from build123d import *

# Parameters (mm, degrees)
SKETCH1_R           = 1
SKETCH1_R_2         = 1.5
BOSS_EXTRUDE1_DEPTH = 3
SKETCH2_R           = 1
CUT_EXTRUDE1_DEPTH  = 10


with BuildPart() as part:
    # Sketch1 → Boss-Extrude1 (new body)
    with BuildSketch(Plane.XY):
        with BuildLine():
            Line((56.489085284, -2.807723586), (56.489085284, -10.511796182))
            ThreePointArc((56.489085284, -10.511796182), (49.919430424, -21.212793876), (37.403860007, -20.196814652))
            ThreePointArc((37.403860007, -20.196814652), (33.591182056, -16.415053625), (31.06380939, -11.676845415))
            ThreePointArc((31.06380939, -11.676845415), (21.265519298, -10.288514848), (12.001109648, -13.767690656))
            ThreePointArc((12.001109648, -13.767690656), (-5.229619348, -14.397609216), (3.208983014, 0.638507613))
            Line((3.208983014, 0.638507613), (53.042854085, 0.638507613))
            ThreePointArc((53.042854085, 0.638507613), (58.925938734, 3.075361063), (56.489085284, -2.807723586))
        make_face()
        with Locations((56.398708828, 0.638507613)):
            Circle(SKETCH1_R, mode=Mode.SUBTRACT)
        with Locations((44.489085284, -10.511796182)):
            Circle(SKETCH1_R_2, mode=Mode.SUBTRACT)
        with Locations((3.208983014, -10.169286947)):
            Circle(SKETCH1_R_2, mode=Mode.SUBTRACT)
        with BuildLine():
            ThreePointArc((38.989085284, -10.511796182), (40.749804307, -14.545129515), (44.90464084, -15.996074947))
            ThreePointArc((44.90464084, -15.996074947), (45.977337989, -16.917660986), (45.055751951, -17.990358135))
            ThreePointArc((45.055751951, -17.990358135), (39.39006577, -16.011796182), (36.989085284, -10.511796182))
            ThreePointArc((36.989085284, -10.511796182), (37.989085284, -9.511796182), (38.989085284, -10.511796182))
        make_face(mode=Mode.SUBTRACT)
        with BuildLine():
            ThreePointArc((6.641982325, -5.872251255), (1.667062363, -4.889847516), (-1.99710038, -8.395394139))
            ThreePointArc((-1.99710038, -8.395394139), (-3.266186962, -9.019428792), (-3.890221615, -7.75034221))
            ThreePointArc((-3.890221615, -7.75034221), (1.106363944, -2.970051359), (7.890345711, -4.309692822))
            ThreePointArc((7.890345711, -4.309692822), (8.047443234, -5.715153732), (6.641982325, -5.872251255))
        make_face(mode=Mode.SUBTRACT)
    extrude(amount=BOSS_EXTRUDE1_DEPTH)

    # Sketch2 → Cut-Extrude1 (cut)
    with BuildSketch(Plane.XY.offset(3)):
        with Locations((0.801619135, -16.035407907)):
            Circle(SKETCH2_R)
    extrude(amount=-CUT_EXTRUDE1_DEPTH, mode=Mode.SUBTRACT)


solid = part.part
Can you work these out from the model? Positions are in its coordinate system, mm. A direction names the side the tool comes from. Give positions to 0.01 mm unless a question says otherwise; leave off trailing zeros. Order: outer loops, then holes, each group sorted by start corner. A loop starts at its lowest first (then second) coordinate and runs counter-clockwise, first axis right, second up. Notation, with made-up numbers: M 19,-16 L 57,-16 A30 cw 57,6 Z; hole C 38,-35.75 d6. An arc over 180 degrees is marked long. Use one line per item in the form item = value.
Item 1: If I drill on line 1 along Y through (x, z) = (44.5, 0.25); line 2 along X through (y, z) = (-14.5, 1.15); line 3 along X through (y, z) = (-6, 0.8), over which ranges is the centre line in solid material (lowest first)? Write a range as [from, to].
Values follow:
line_1 = [-22.51, -18.01], [-16.01, -12.01], [-9.01, 0.64]
line_2 = [-5.17, 11.58], [32.35, 38.14], [40.7, 55.81]
line_3 = [-6.13, -3.03], [-0.38, 6.85], [7.68, 56.49]
Item 2: Will these pins go through, and if not, where does the flat tip stop? pin 1 Ø2.5 at (x, y) = (44.49, -10.51) entering from -Z; pin 2 Ø0.9 at (x, z) = (39, 1.5) entering from +Y.
Values follow:
pin_1 = through
pin_2 = 0.64
Item 3: If we section it at B-B, the plane x = 34.5: Write out the boundary of the cut face in (y, z).
Values follow:
outline = M -17.54,0 L 0.64,0 L 0.64,3 L -17.54,3 Z
Item 4: If we section it at C-C, the plane x = 48: Write out the boundary of the cut face in (y, z), and give its area (3 significant figures).
Values follow:
outline = M -21.99,0 L 0.64,0 L 0.64,3 L -21.99,3 Z
area = 67.9 mm^2
Item 5: Thinking about a two-plate mould opening in X: for faces 1 (the cylindrical face through (2.884, -11.634, 1.479)), 2 (the cylindrical face through (50.08, -21.13, 1.48)), 3 (the flat face through (27, -9, 3)), which applies, pulls with the +X half, pulls with the -X half, needs draft (parallel to the pull), parting line crosses it, or undercut?
Values follow:
face_1 = undercut
face_2 = parting line crosses it
face_3 = needs draft
Item 6: For faces 4 (the cylindrical face through (1, -3, 1)), 5 (the flat face through (56.489, -7, 1)), 6 (the flat face through (28, 0.639, 1)), which set-ups out of +Z, -Z, +X, -X, +Y, -Y let a thin tool reach every point of the face, with its end or its side?
Values follow:
face_4 = +Z, -Z
face_5 = +Z, -Z, +X, -Y
face_6 = +Z, -Z, -X, +Y
Item 7: If we section it at A-A, the plane z = 1.45: Write out the boundary of the cut face in (x, y), and give its area (3 significant figures).
Values follow:
outline = M 3.21,0.64 A9.89 ccw long 12,-13.77 A20 cw 31.06,-11.68 A18 ccw 37.4,-20.2 A12 ccw 56.49,-10.51 L 56.49,-2.81 A3.45 ccw long 53.04,0.64 Z; hole M -3.89,-7.75 A1 ccw -2,-8.4 A5.5 cw 6.64,-5.87 A1 ccw 7.89,-4.31 A7.5 ccw Z; hole C 0.8,-16.04 d2; hole C 3.21,-10.17 d3; hole M 36.99,-10.51 A7.5 ccw 45.06,-17.99 A1 ccw 44.9,-16 A5.5 cw 38.99,-10.51 A1 ccw Z; hole C 44.49,-10.51 d3; hole C 56.4,0.64 d2
area = 1,010 mm^2
